```python
from build123d import *

# Parameters (mm, degrees)
Y_KSEKLIK_EKSTR_ZYON1_DEPTH = 20
CUT_EXTRUDE1_DEPTH          = 44
CUT_EXTRUDE1_DEPTH_BACK     = 10
SKETCH1_R                   = 2.5
SKETCH2_W                   = 32
SKETCH2_H                   = 30
CUT_EXTRUDE3_DEPTH          = 27
SKETCH3_W                   = 32
SKETCH3_H                   = 30
BOSS_EXTRUDE1_DEPTH         = 16
CUT_EXTRUDE4_DEPTH          = 4
SKETCH5_W                   = 33.515954684
SKETCH5_H                   = 18.308274805
BOSS_EXTRUDE2_DEPTH         = 10
CUT_EXTRUDE5_DEPTH          = 53
CUT_EXTRUDE5_DEPTH_BACK     = 25
SKETCH6_R                   = 2.5
SKETCH7_W                   = 36.495036791
SKETCH7_H                   = 91.485439351
SKETCH7_W_2                 = 38.306268879
CUT_EXTRUDE7_DEPTH          = 30
SKETCH8_W                   = 29
SKETCH8_H                   = 90
BOSS_EXTRUDE3_DEPTH         = 10
CUT_EXTRUDE8_DEPTH          = 10
SKETCH10_W                  = 32
SKETCH10_H                  = 30
CUT_EXTRUDE9_DEPTH          = 28
SKETCH11_W                  = 32
SKETCH11_H                  = 30
BOSS_EXTRUDE4_DEPTH         = 10
SKETCH12_R                  = 3
CUT_EXTRUDE10_DEPTH         = 22
SKETCH13_R                  = 6
CUT_EXTRUDE11_DEPTH         = 5
FILLET1_R                   = 1.5


with BuildPart() as part:
    # Çizim1 → Yükseklik-Ekstrüzyon1 (new body)
    with BuildSketch(Plane.XY):
        with BuildLine():
            Line((-41.541366964, -1.110887656), (-41.541366964, 48.889112344))
            ThreePointArc((-41.541366964, 48.889112344), (-35.683502588, 63.031247968), (-21.541366964, 68.889112344))
            Line((-21.541366964, 68.889112344), (28.458633036, 68.889112344))
            ThreePointArc((28.458633036, 68.889112344), (42.600768659, 63.031247968), (48.458633036, 48.889112344))
            Line((48.458633036, 48.889112344), (48.458633036, -1.110887656))
            ThreePointArc((48.458633036, -1.110887656), (42.600768659, -15.25302328), (28.458633036, -21.110887656))
            Line((28.458633036, -21.110887656), (-21.541366964, -21.110887656))
            ThreePointArc((-21.541366964, -21.110887656), (-35.683502588, -15.25302328), (-41.541366964, -1.110887656))
        make_face()
    extrude(amount=Y_KSEKLIK_EKSTR_ZYON1_DEPTH)

    # Sketch1 → Cut-Extrude1 (cut, two sides: drawn at the far end of the back side and taken through both)
    with BuildSketch(Plane.XY.offset(-CUT_EXTRUDE1_DEPTH_BACK)):
        with Locations(Location((-4.041366964, 23.889112344, 0), (0, 0, 180))):
            Circle(SKETCH1_R)
        with Locations(Location((10.958633036, 23.889112344, 0), (0, 0, 180))):
            Circle(SKETCH1_R)
    extrude(amount=CUT_EXTRUDE1_DEPTH + CUT_EXTRUDE1_DEPTH_BACK, mode=Mode.SUBTRACT)

    # Sketch2 → Cut-Extrude3 (cut)
    with BuildSketch(Plane.XY):
        with Locations((3.458633036, 53.889112344)):
            Rectangle(SKETCH2_W, SKETCH2_H)
    extrude(amount=CUT_EXTRUDE3_DEPTH, mode=Mode.SUBTRACT)

    # Sketch3 → Boss-Extrude1 (add)
    with BuildSketch(Plane.XY):
        with Locations((3.458633036, 53.889112344)):
            Rectangle(SKETCH3_W, SKETCH3_H)
    extrude(amount=BOSS_EXTRUDE1_DEPTH)

    # Sketch4 → Cut-Extrude4 (cut)
    with BuildSketch(Plane.XY):
        Polygon((15.692905243, 23.889112344), (13.325769139, 27.989112344), (8.591496932, 27.989112344), (6.224360828, 23.889112344), (8.591496932, 19.789112344), (13.325769139, 19.789112344), align=None)
        Polygon((0.692905243, 23.889112344), (-1.674230861, 27.989112344), (-6.408503068, 27.989112344), (-8.775639172, 23.889112344), (-6.408503068, 19.789112344), (-1.674230861, 19.789112344), align=None)
    extrude(amount=CUT_EXTRUDE4_DEPTH, mode=Mode.SUBTRACT)

    # Sketch5 → Boss-Extrude2 (add)
    with BuildSketch(Plane.XY):
        with Locations((2.203630327, 23.667641278)):
            Rectangle(SKETCH5_W, SKETCH5_H)
    extrude(amount=BOSS_EXTRUDE2_DEPTH)

    # Sketch6 → Cut-Extrude5 (cut, two sides: drawn at the far end of the back side and taken through both)
    with BuildSketch(Plane.XY.offset(-CUT_EXTRUDE5_DEPTH_BACK)):
        with Locations(Location((-4.041366964, 23.889112344, 0), (0, 0, 180))):
            Circle(SKETCH6_R)
        with Locations(Location((10.958633036, 23.889112344, 0), (0, 0, 180))):
            Circle(SKETCH6_R)
    extrude(amount=CUT_EXTRUDE5_DEPTH + CUT_EXTRUDE5_DEPTH_BACK, mode=Mode.SUBTRACT)

    # Sketch7 → Cut-Extrude7 (cut)
    with BuildSketch(Plane.XY):
        with Locations((-30.78888536, 23.146392668)):
            Rectangle(SKETCH7_W, SKETCH7_H)
        with Locations((38.611767476, 23.146392668)):
            Rectangle(SKETCH7_W_2, SKETCH7_H)
    extrude(amount=CUT_EXTRUDE7_DEPTH, mode=Mode.SUBTRACT)

    # Sketch8 → Boss-Extrude3 (add)
    with BuildSketch(Plane.XY):
        with Locations((-27.041366964, 23.889112344)):
            Rectangle(SKETCH8_W, SKETCH8_H)
        with Locations((33.958633036, 23.889112344)):
            Rectangle(SKETCH8_W, SKETCH8_H)
    extrude(amount=BOSS_EXTRUDE3_DEPTH)

    # Sketch9 → Cut-Extrude8 (cut)
    with BuildSketch(Plane.XY):
        with BuildLine():
            Line((-41.541366964, 68.889112344), (-21.541366964, 68.889112344))
            ThreePointArc((-21.541366964, 68.889112344), (-35.683502588, 63.031247968), (-41.541366964, 48.889112344))
            Line((-41.541366964, 48.889112344), (-41.541366964, 68.889112344))
        make_face()
        with BuildLine():
            Line((48.458633036, 68.889112344), (48.458633036, 48.889112344))
            ThreePointArc((48.458633036, 48.889112344), (42.600768659, 63.031247968), (28.458633036, 68.889112344))
            Line((28.458633036, 68.889112344), (48.458633036, 68.889112344))
        make_face()
        with BuildLine():
            Line((48.458633036, -21.110887656), (28.458633036, -21.110887656))
            ThreePointArc((28.458633036, -21.110887656), (42.600768659, -15.25302328), (48.458633036, -1.110887656))
            Line((48.458633036, -1.110887656), (48.458633036, -21.110887656))
        make_face()
        with BuildLine():
            Line((-41.541366964, -21.110887656), (-41.541366964, -1.110887656))
            ThreePointArc((-41.541366964, -1.110887656), (-35.683502588, -15.25302328), (-21.541366964, -21.110887656))
            Line((-21.541366964, -21.110887656), (-41.541366964, -21.110887656))
        make_face()
    extrude(amount=CUT_EXTRUDE8_DEPTH, mode=Mode.SUBTRACT)

    # Sketch10 → Cut-Extrude9 (cut)
    with BuildSketch(Plane.XY):
        with Locations((3.458633036, 53.889112344)):
            Rectangle(SKETCH10_W, SKETCH10_H)
        with Locations((3.458633036, -6.110887656)):
            Rectangle(SKETCH10_W, SKETCH10_H)
    extrude(amount=CUT_EXTRUDE9_DEPTH, mode=Mode.SUBTRACT)

    # Sketch11 → Boss-Extrude4 (add)
    with BuildSketch(Plane.XY):
        with Locations((3.458633036, 53.889112344)):
            Rectangle(SKETCH11_W, SKETCH11_H)
        with Locations((3.458633036, -6.110887656)):
            Rectangle(SKETCH11_W, SKETCH11_H)
    extrude(amount=BOSS_EXTRUDE4_DEPTH)

    # Sketch12 → Cut-Extrude10 (cut)
    with BuildSketch(Plane.XY):
        with Locations(Location((-4.041366964, 23.889112344, 0), (0, 0, 180))):
            Circle(SKETCH12_R)
        with Locations(Location((10.958633036, 23.889112344, 0), (0, 0, 180))):
            Circle(SKETCH12_R)
    extrude(amount=CUT_EXTRUDE10_DEPTH, mode=Mode.SUBTRACT)

    # Sketch13 → Cut-Extrude11 (cut)
    with BuildSketch(Plane.XY):
        with Locations((10.958633036, 23.889112344)):
            Circle(SKETCH13_R)
        with Locations((-4.041366964, 23.889112344)):
            Circle(SKETCH13_R)
    extrude(amount=CUT_EXTRUDE11_DEPTH, mode=Mode.SUBTRACT)

    # Fillet1
    fillet1_edges = [part.edges().sort_by_distance(p)[0] for p in [
        (-41.541366964, 23.889112344, 0),
        (-35.683502588, 63.031247968, 0),
        (3.458633036, 68.889112344, 0),
        (42.600768659, 63.031247968, 0),
        (48.458633036, 23.889112344, 0),
        (42.600768659, -15.25302328, 0),
        (3.458633036, -21.110887656, 0),
        (-35.683502588, -15.25302328, 0),
    ]]
    fillet(fillet1_edges, radius=FILLET1_R)


solid = part.part
```
Work out the finished part from the listing and answer in its coordinate system (mm). A direction names the side the tool comes from. Give positions to 0.01 mm unless a question says otherwise; leave off trailing zeros. Order: outer loops, then holes, each group sorted by start corner. A loop starts at its lowest first (then second) coordinate and runs counter-clockwise, first axis right, second up. Notation, with made-up numbers: M 89,65.5 L 116,65.5 A32 ccw 116,104.5 Z; hole C 53.25,45 d5. An arc over 180 degrees is marked long. Return JSON: item names as keys, results as strings.
1) Section A-A, the plane y = 45.5 is taken. Write down the section's boundary in (x, z).
Resolved:
{"outline": "M -41.54,1.5 A1.5 ccw -40.04,0 L 46.96,0 A1.5 ccw 48.46,1.5 L 48.46,10 L -41.54,10 Z"}
2) Straight lines are drawn through the part: line 1 along Z through (x, y) = (-4, 49); line 2 along Y through (x, z) = (9, 12); line 3 along X through (y, z) = (27, 19). For each, find the intervals that lie inside material, in ascending order. Write a range as [from, to].
Resolved:
{"line 1": "[0, 10]", "line 2": "[8.89, 21.62], [26.16, 38.89]", "line 3": "[-12.54, 19.46]"}
3) A tool of negligible diameter and unlimited length cuts with its end or side. For faces 1 (the cylindrical face through (9.66, 18.03, 2.46)), 2 (the flat face through (19.459, 24, 15)), 3 (the flat face through (3, 8.889, 15)), 4 (the flat face through (3, 38.889, 15)), from which of +Z, -Z, +X, -X, +Y, -Y can it reach the whole face along a straight path? Write none if from no direction.
Resolved:
{"face 1": "-Z", "face 2": "+Z, +X, +Y, -Y", "face 3": "+Z, +X, -X, -Y", "face 4": "+Z, +X, -X, +Y"}
4) Each of these flat-tipped pins is pushed along its axis until it touches: pin 1 (13 mm diameter, centred on x = 9, y = 23.5, fed in from -Z); pin 2 (3 mm diameter, centred on y = 30.5, z = 16, fed in from +X); pin 3 (4 mm diameter, centred on y = 51, z = 12.5, fed in from -X); pin 4 (9.5 mm diameter, centred on x = 10.96, y = 23.89, fed in from -Z). Where does it stop, or does it pass through?
Resolved:
{"pin 1": "z = 0", "pin 2": "x = 19.46", "pin 3": "through", "pin 4": "z = 5"}
5) For a pull along X with two mould halves and no side action, classify faces 5 (the flat face through (3, 24, 0)), 6 (the cylindrical face through (-5.34, 18.03, 2.46)), 7 (the cylindrical face through (42.76, 62.87, 5.69)) as +X half, -X half, draft (parallel to the pull), parting line (faces both ways), or undercut.
Resolved:
{"face 5": "draft", "face 6": "undercut", "face 7": "+X half"}
6) Section C-C, the plane x = -17 is taken. Write down the section's boundary in (y, z).
Resolved:
{"outline": "M -21.11,1.5 A1.5 ccw -19.61,0 L 67.39,0 A1.5 ccw 68.89,1.5 L 68.89,10 L -21.11,10 Z"}
7) Section B-B, the plane z = 3.5 is taken. Write down the section's boundary in (x, y).
Resolved:
{"outline": "M -41.54,-1.11 A20 ccw -21.54,-21.11 L 28.46,-21.11 A20 ccw 48.46,-1.11 L 48.46,48.89 A20 ccw 28.46,68.89 L -21.54,68.89 A20 ccw -41.54,48.89 Z; hole C -4.04,23.89 d12; hole C 10.96,23.89 d12"}
8) Section D-D, the plane y = 16 is taken. Write down the section's boundary in (x, z).
Resolved:
{"outline": "M -41.54,1.5 A1.5 ccw -40.04,0 L 46.96,0 A1.5 ccw 48.46,1.5 L 48.46,10 L 19.46,10 L 19.46,20 L -12.54,20 L -12.54,10 L -41.54,10 Z"}
